For this review, take the finished solid that the model builds, in its own axes (mm). Face numbers are marked on the shaded views. A direction names the side the tool comes from. Give positions to 0.01 mm unless a question says otherwise; leave off trailing zeros. Order: outer loops, then holes, each group sorted by start corner. A loop starts at its lowest first (then second) coordinate and runs counter-clockwise, first axis right, second up. Notation, with made-up numbers: (2.5, -38.75) - (51.5, -38.75) arc R12 ccw to (51.5, -28.75) - close; hole circle Ø1 at (22, 71.5). An arc over 180 degrees is marked (long way). One line per item, written item: value.
```python
from build123d import *

# Parameters (mm, degrees)
F0_W     = 12.7
F0_H     = 50.8
F1_DEPTH = 25.4
F2_DEPTH = 12.7
F3_W     = 19.05
F3_H     = 25.4
F4_DEPTH = 50.8


with BuildPart() as f1:
    # F0 (on Front) → F1 (new body, symmetric)
    with BuildSketch(Plane.XZ):
        with Locations((6.35, 25.4)):
            Rectangle(F0_W, F0_H)
        Polygon((12.7, 50.8), (12.7, 0), (38.1, 0), (38.1, 29.028575), align=None)
    extrude(amount=F1_DEPTH, both=True)

    # F0 (on Front) → F2 (join, symmetric)
    with BuildSketch(Plane.XZ):
        with Locations((-6.35, 25.4)):
            Rectangle(F0_W, F0_H)
    extrude(amount=F2_DEPTH, both=True)

    # F3 (on Top) → F4 (cut)
    with BuildSketch(Plane.XY):
        with Locations((28.575, 0)):
            Rectangle(F3_W, F3_H)
    extrude(amount=F4_DEPTH, mode=Mode.SUBTRACT)


solid = f1.part
```
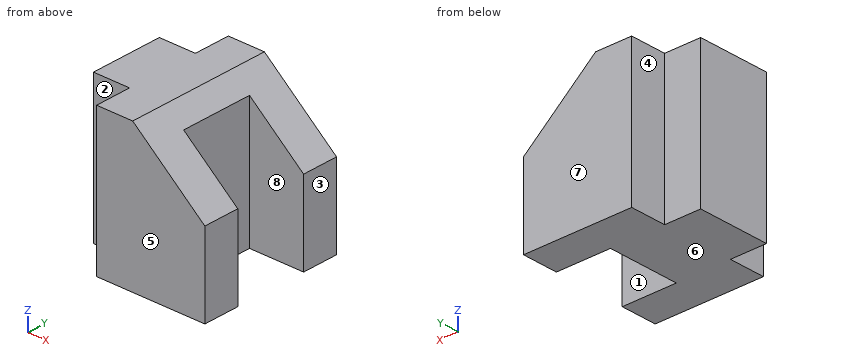
(1) Take a section at D-D (x = 20). Write out the cut boundary in (y, z), then the cut area to 3 significant figures.
Answers below:
outline: (-25.4, 0) - (-12.7, 0) - (-12.7, 44.54) - (-25.4, 44.54) - close; (12.7, 0) - (25.4, 0) - (25.4, 44.54) - (12.7, 44.54) - close
area: 1,130 mm^2
(2) Take a section at B-B (z = 16.5). Write out the cut boundary in (x, y), then the cut area to 3 significant figures.
Answers below:
outline: (-12.7, -12.7) - (0, -12.7) - (0, -25.4) - (38.1, -25.4) - (38.1, -12.7) - (19.05, -12.7) - (19.05, 12.7) - (38.1, 12.7) - (38.1, 25.4) - (0, 25.4) - (0, 12.7) - (-12.7, 12.7) - close
area: 1,770 mm^2
(3) Wall thickness on line 1 (Y direction, x = 35.5, z = 21); line 2 (X direction, y = 19.5, z = 16.5); line 3 (Y direction, x = -1, z = 45.5): over which ranges is each line inside the solid? List them lowest first. Write a range as from..to.
Answers below:
line 1: y = -25.4..-12.7, 12.7..25.4
line 2: x = 0..38.1
line 3: y = -12.7..12.7
(4) Take a section at A-A (x = 33). Write out the cut boundary in (y, z), then the cut area to 3 significant figures.
Answers below:
outline: (-25.4, 0) - (-12.7, 0) - (-12.7, 33.4) - (-25.4, 33.4) - close; (12.7, 0) - (25.4, 0) - (25.4, 33.4) - (12.7, 33.4) - close
area: 848 mm^2
(5) For P1, Ø6.5, axis at y = 20.5, z = 13, coming from the -X side; P2, Ø12, axis at x = 25.5, y = 3, coming from the +Z side; P3, Ø12.5, axis at y = -2, z = 15.5, coming from the +X side; P4, Ø14, axis at x = -9.5, z = 19, coming from the -Y side, all flat-tipped, find the tip position at first contact; note any pin that passes through.
Answers below:
P1: stops at x = 0
P2: passes through
P3: stops at x = 19.05
P4: stops at y = -12.7
(6) Take a section at C-C (y = -7). Write out the cut boundary in (x, z).
Answers below:
outline: (-12.7, 0) - (19.05, 0) - (19.05, 45.36) - (12.7, 50.8) - (-12.7, 50.8) - close
(7) Machinability: for the marked faces 1, 2, 3 and 4, which of the approach directions +Z, -Z, +X, -X, +Y, -Y give a long, thin tool a straight path to every point of the face, cutting with its end or side? Answer none if there is none.
Answers below:
face 1: +Z, -Z, +X
face 2: +Z, -Z, -X, -Y
face 3: +Z, -Z, +X, +Y, -Y
face 4: +Z, -Z, -X, +Y
(8) Draft analysis for pull direction Y (two halves, no side actions). For the marked faces 5, 6, 7 and 8, state which applies: pulls with the +Y half, pulls with the -Y half, needs draft (parallel to the pull), parting line crosses it, or undercut.
Answers below:
face 5: pulls with the -Y half
face 6: needs draft
face 7: pulls with the +Y half
face 8: undercut
